from build123d import *

# Parameters (mm, degrees)
SKETCH1_W           = 90
SKETCH1_H           = 46
BOSS_EXTRUDE1_DEPTH = 3
SKETCH5_R           = 1.5
CUT_EXTRUDE3_DEPTH  = 4
SKETCH6_W           = 2
SKETCH6_H           = 28
SKETCH6_W_2         = 60
SKETCH6_H_2         = 2
SKETCH6_H_3         = 3
SKETCH6_W_3         = 45
BOSS_EXTRUDE3_DEPTH = 20
SKETCH7_R           = 1.5
CUT_EXTRUDE4_DEPTH  = 4
SKETCH8_R           = 3
CUT_EXTRUDE5_DEPTH  = 2.1
SKETCH9_W           = 2
SKETCH9_H           = 11
SKETCH9_W_2         = 20
SKETCH9_H_2         = 2
SKETCH9_W_3         = 1
SKETCH9_H_3         = 42
BOSS_EXTRUDE4_DEPTH = 6


with BuildPart() as part:
    # Sketch1 → Boss-Extrude1 (new body)
    with BuildSketch(Plane(origin=(0, 0, 0), x_dir=(1, 0, 0), z_dir=(0, 1, 0))):
        with Locations((-15.229105331, -10.267137121)):
            Rectangle(SKETCH1_W, SKETCH1_H)
    extrude(amount=BOSS_EXTRUDE1_DEPTH)

    # Sketch5 → Cut-Extrude3 (cut, through all)
    with BuildSketch(Plane(origin=(0, 3, 0), x_dir=(1, 0, 0), z_dir=(0, 1, 0))):
        with Locations((-57.229105331, -22.267137121)):
            Circle(SKETCH5_R)
        with Locations((-57.229105331, 1.732862879)):
            Circle(SKETCH5_R)
        with Locations((0.770894669, -10.267137121)):
            Circle(SKETCH5_R)
    extrude(amount=-CUT_EXTRUDE3_DEPTH, mode=Mode.SUBTRACT)

    # Sketch6 → Boss-Extrude3 (add)
    with BuildSketch(Plane(origin=(0, 3, 0), x_dir=(1, 0, 0), z_dir=(0, 1, 0))):
        with Locations((28.770894669, -17.267137121)):
            Rectangle(SKETCH6_W, SKETCH6_H)
        Polygon((29.770894669, -31.267137121), (27.770894669, -31.267137121), (4.770894669, -31.267137121), (4.770894669, -33.267137121), (29.770894669, -33.267137121), align=None)
        with Locations((-25.229105331, -32.267137121)):
            Rectangle(SKETCH6_W_2, SKETCH6_H_2)
        with Locations((28.770894669, 9.232862879)):
            Rectangle(SKETCH6_W, SKETCH6_H_3)
        Polygon((9.770894669, 10.732862879), (27.770894669, 10.732862879), (29.770894669, 10.732862879), (29.770894669, 12.732862879), (9.770894669, 12.732862879), align=None)
        with Locations((-32.729105331, 11.732862879)):
            Rectangle(SKETCH6_W_3, SKETCH6_H_2)
    extrude(amount=BOSS_EXTRUDE3_DEPTH)

    # Sketch7 → Cut-Extrude4 (cut, through all)
    with BuildSketch(Plane(origin=(0, 3, 0), x_dir=(1, 0, 0), z_dir=(0, 1, 0))):
        with Locations((15.770894669, -26.267137121)):
            Circle(SKETCH7_R)
        with Locations((-44.229105331, -26.267137121)):
            Circle(SKETCH7_R)
        with Locations((15.770894669, 5.732862879)):
            Circle(SKETCH7_R)
        with Locations((-44.229105331, 5.732862879)):
            Circle(SKETCH7_R)
    extrude(amount=-CUT_EXTRUDE4_DEPTH, mode=Mode.SUBTRACT)

    # Sketch8 → Cut-Extrude5 (cut)
    with BuildSketch(Plane(origin=(0, 0, 0), x_dir=(-1, 0, 0), z_dir=(0, -1, 0))):
        with Locations((-15.770894669, -26.267137121)):
            Circle(SKETCH8_R)
        with Locations((-15.770894669, 5.732862879)):
            Circle(SKETCH8_R)
        with Locations((44.229105331, -26.267137121)):
            Circle(SKETCH8_R)
        with Locations((44.229105331, 5.732862879)):
            Circle(SKETCH8_R)
    extrude(amount=-CUT_EXTRUDE5_DEPTH, mode=Mode.SUBTRACT)

    # Sketch9 → Boss-Extrude4 (add)
    with BuildSketch(Plane(origin=(0, 3, 0), x_dir=(1, 0, 0), z_dir=(0, 1, 0))):
        with Locations((28.770894669, 2.232862879)):
            Rectangle(SKETCH9_W, SKETCH9_H)
        with Locations((-0.229105331, 11.732862879)):
            Rectangle(SKETCH9_W_2, SKETCH9_H_2)
        with Locations((-54.729105331, -10.267137121)):
            Rectangle(SKETCH9_W_3, SKETCH9_H_3)
    extrude(amount=BOSS_EXTRUDE4_DEPTH)


solid = part.part
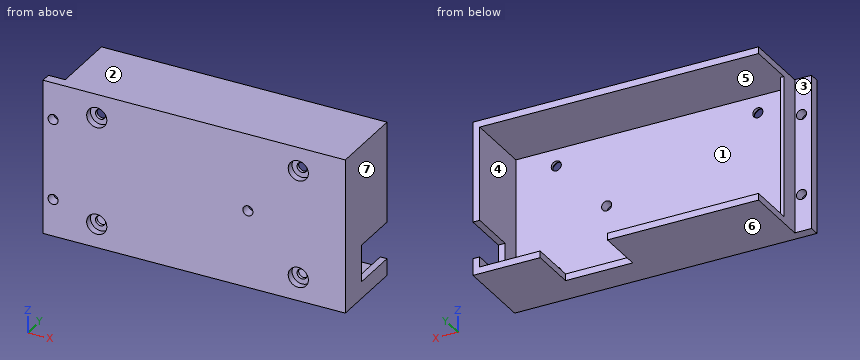
Design review of the part built by this model. Coordinates are the model's own, in mm. Face numbers are marked on the shaded views. A direction names the side the tool comes from. Coordinates: 2 decimals unless noted, no trailing zeros. Order: outer loops, then holes, each group sorted by start corner. A loop starts at its lowest first (then second) coordinate and runs counter-clockwise, first axis right, second up. Notation, with made-up numbers: (25.5, 8.25) -> (74.5, 8.25) arc R24 cw to (74.5, 38.25) -> close; hole circle Ø4 at (3, -35.75). An arc over 180 degrees is marked (long way). Use one line per item in the form item = value. Start each with the question number.
(1) Add section A-A on y = 13. State the section outline as (x, z) points, plus the area to 3 significant figures.
(2) For the marked faces 1, 2 and 3, list the 3-axis set-ups (+Z, -Z, +X, -X, +Y, -Y) from which the entire face can be reached by the end or side of a thin tool; tool diameter is ignored.
(3) Add section D-D on z = 5. State the section outline as (x, y) points.
(4) Insertion check: pin 1 (21 mm diameter, centred on x = 1.5, z = 13, fed in from +Y); pin 2 (1.5 mm diameter, centred on x = 17.5, z = -3, fed in from -Y); pin 3 (1.1 mm diameter, centred on x = -55, z = 9, fed in from +Y); pin 4 (5 mm diameter, centred on x = 15.77, z = -5.73, fed in from -Y). Each pin has a flat end and moves straight along its axis. Give the tip position at first contact, or say it passes through.
(5) Add section C-C on y = 6.25. State the section outline as (x, z) points, plus the area to 3 significant figures.
(6) The part is to be moulded in two halves that separate along X. For the marked faces 4, 5, 6 and 7, say which applies: +X half, -X half, draft (parallel to the pull), parting line (faces both ways), or undercut.
(7) For probe 1 along X at (y, z) = (4.25, 12.5); probe 2 along Z at (x, y) = (-52.5, 12); probe 3 along X at (y, z) = (17, 27), list the stretches that pass through material, from the lowest coordinate up.
(8) Add section B-B on x = -51. State the section outline as (y, z) points.
Answer block:
q1.outline = (-55.23, -12.73) -> (-10.23, -12.73) -> (-10.23, -10.73) -> (-55.23, -10.73) -> close; (-55.23, 31.27) -> (27.77, 31.27) -> (27.77, 3.27) -> (29.77, 3.27) -> (29.77, 33.27) -> (-55.23, 33.27) -> close; (9.77, -12.73) -> (29.77, -12.73) -> (29.77, -7.73) -> (27.77, -7.73) -> (27.77, -10.73) -> (9.77, -10.73) -> close
q1.area = 362 mm²
q2.face_1 = +Y
q2.face_2 = +Z, +X, -X, +Y, -Y
q2.face_3 = +Z, -Z, -X, +Y
q3.outline = (-60.23, 0) -> (29.77, 0) -> (29.77, 23) -> (27.77, 23) -> (27.77, 3) -> (-54.23, 3) -> (-54.23, 9) -> (-55.23, 9) -> (-55.23, 3) -> (-60.23, 3) -> close
q4.pin_1 = 3
q4.pin_2 = 0
q4.pin_3 = 9
q4.pin_4 = 2.1
q5.outline = (-55.23, -12.73) -> (29.77, -12.73) -> (29.77, 33.27) -> (-55.23, 33.27) -> close; hole (-54.23, -10.73) -> (27.77, -10.73) -> (27.77, 31.27) -> (-54.23, 31.27) -> close
q5.area = 466 mm²
q6.face_4 = undercut
q6.face_5 = undercut
q6.face_6 = draft
q6.face_7 = +X half
q7.probe_1 = -55.23 to -54.23, 27.77 to 29.77
q7.probe_2 = -12.73 to -10.73, 31.27 to 33.27
q7.probe_3 = 27.77 to 29.77
q8.outline = (0, -12.73) -> (23, -12.73) -> (23, -10.73) -> (3, -10.73) -> (3, 31.27) -> (23, 31.27) -> (23, 33.27) -> (0, 33.27) -> close
